from build123d import *

# Parameters (mm, degrees)
SKETCH001_R     = 3.75
POCKET_DEPTH    = 9.70192
CHAMFER_SIZE    = 0.4
CHAMFER001_SIZE = 0.1


with BuildPart() as pocket:
    # Sketch003 → Revolution001 (revolve)
    with BuildSketch(Plane.XZ):
        Polygon((0, 0.29908), (2.75, 1.3), (2.75, 10), (0, 10), align=None)
    revolve(axis=Axis((0, 0, 0), (0, 0, 1)))

    # Sketch001 → Pocket (cut, through all)
    with BuildSketch(Plane(origin=(0, 0, 10), x_dir=(-1, 0, 0), z_dir=(0, 0, 1))):
        Circle(SKETCH001_R)
        Polygon((-0.721688, 1.25), (0.721688, 1.25), (1.443376, 0), (0.721688, -1.25), (-0.721688, -1.25), (-1.443376, 0), align=None, mode=Mode.SUBTRACT)
    extrude(amount=-POCKET_DEPTH, mode=Mode.SUBTRACT)


with BuildPart() as chamfer001:
    # Sketch → Revolution (revolve)
    with BuildSketch(Plane.XZ):
        Polygon((1.45, 3), (2.75, 3), (2.75, 0), (1.5, 0), (1.5, -18), (0, -18), (0, 1.549999), align=None)
    revolve(axis=Axis((0, 0, 0), (0, 0, 1)))

    # Cut: cut Pocket
    add(pocket.part, mode=Mode.SUBTRACT)

    # Chamfer
    chamfer_edges = [chamfer001.edges().sort_by_distance(p)[0] for p in [
        (-1.5, 0, -18),
    ]]
    chamfer(chamfer_edges, length=CHAMFER_SIZE)

    # Chamfer001
    chamfer001_edges = [chamfer001.edges().sort_by_distance(p)[0] for p in [
        (-2.75, 0, 0),
        (-2.75, 0, 3),
    ]]
    chamfer(chamfer001_edges, length=CHAMFER001_SIZE)


solid = chamfer001.part
CAD build for the part. Positions are in the model's coordinates, mm. A direction names the side the tool comes from. Give positions to 0.01 mm unless a question says otherwise; leave off trailing zeros. Order: outer loops, then holes, each group sorted by start corner. A loop starts at its lowest first (then second) coordinate and runs counter-clockwise, first axis right, second up. Notation, with made-up numbers: (21.25, 71) -> (45.25, 71) arc R25 ccw to (45.25, 100) -> close; hole circle Ø4 at (30.5, 88). An arc over 180 degrees is marked (long way). Return JSON: item names as keys, results as strings.
Q1. Saw through at A-A (z = -15.5). Write the cut outline in (x, y).
Working result:
{"outline": "circle Ø3 at (0, 0)"}
Q2. Which spindle directions (+Z, -Z, +X, -X, +Y, -Y) get a long thin tool onto all of the face, cutting with end or side? Do faces 4 (the face through (-1.088, 0.616, 1.889)), 5 (the face through (0, 0, -18)). Say none if no direction does.
Working result:
{"face 4": "+Z", "face 5": "-Z, +X, -X, +Y, -Y"}
Q3. Mould opens along Y. For faces 1 (the face through (0, -2, 0)), 2 (the face through (-0.067, 0.061, 0.332)), 3 (the face through (-1.5, 0.07, -8.92)) say: pulls with the +Y half, pulls with the -Y half, needs draft (parallel to the pull), parting line crosses it, or undercut.
Working result:
{"face 1": "needs draft", "face 2": "undercut", "face 3": "parting line crosses it"}
Q4. Flat gauge pins, fed straight in: pin 1 (1.5 mm diameter, centred on x = 0.5, z = -14, fed in from -Y); pin 2 (2 mm diameter, centred on y = -1.5, z = -10.5, fed in from -X); pin 3 (1.5 mm diameter, centred on x = 0.5, y = 0, fed in from +Z). Where does each tip first touch, or does it go through?
Working result:
{"pin 1": "y = -1.5", "pin 2": "x = -1.41", "pin 3": "z = 0.75"}
Q5. Drill centre lines: line 1 (Z direction, x = -0.85, y = -1.55); line 2 (X direction, y = -0.6, z = -6); line 3 (X direction, y = -0.85, z = -2.75). Where is each one in solid material? Low to high.
Working result:
{"line 1": "0 to 3", "line 2": "-1.37 to 1.37", "line 3": "-1.24 to 1.24"}
